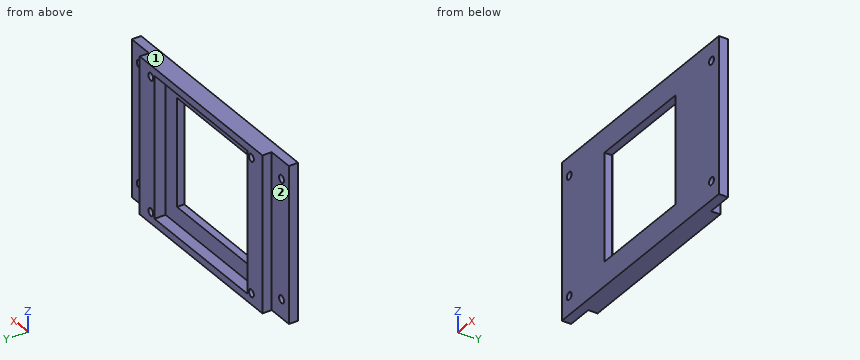
```python
from build123d import *

# Parameters (mm, degrees)
SKETCH1_R            = 11
SKETCH1_R_2          = 7.5
EXTRUDE_THIN1_DEPTH  = 10
BOSS_EXTRUDE2_DEPTH  = 10
SKETCH6_W            = 10
SKETCH6_H            = 5
BOSS_EXTRUDE3_DEPTH  = 10
SKETCH8_W            = 10
SKETCH8_H            = 5
BOSS_EXTRUDE4_DEPTH  = 10
SKETCH9_W            = 42
SKETCH9_H            = 5
BOSS_EXTRUDE5_DEPTH  = 54
SKETCH19_W           = 38
SKETCH19_H           = 38
CUT_EXTRUDE3_DEPTH   = 3
SKETCH25_W           = 29
SKETCH25_H           = 29
CUT_EXTRUDE4_DEPTH   = 2
SKETCH26_R           = 1.00264766
CUT_EXTRUDE5_DEPTH   = 3
LPATTERN4_COUNT      = 2
LPATTERN4_PITCH      = 36
LPATTERN4_COUNT_DIR2 = 2
LPATTERN4_PITCH_DIR2 = 41
SKETCH29_W           = 22
SKETCH29_H           = 36
CUT_EXTRUDE8_DEPTH   = 10
SKETCH35_R           = 1
CUT_EXTRUDE9_DEPTH   = 5
LPATTERN5_COUNT      = 2
LPATTERN5_PITCH      = 58
LPATTERN5_COUNT_DIR2 = 2
LPATTERN5_PITCH_DIR2 = 32
SKETCH37_W           = 42
SKETCH37_H           = 2.5
CUT_EXTRUDE10_DEPTH  = 5
SKETCH38_W           = 42
SKETCH38_H           = 2.5
CUT_EXTRUDE11_DEPTH  = 5
SKETCH39_W           = 1.998284703
SKETCH39_H           = 42
CUT_EXTRUDE12_DEPTH  = 2.5
SKETCH41_W           = 1.997921913
SKETCH41_H           = 42
CUT_EXTRUDE13_DEPTH  = 2.5


with BuildPart() as part:
    # Sketch1 → Extrude-Thin1 (new body)
    with BuildSketch(Plane(origin=(0, 0, 0), x_dir=(0, 0, -1), z_dir=(1, 0, 0))):
        Circle(SKETCH1_R)
        Circle(SKETCH1_R_2, mode=Mode.SUBTRACT)
    extrude(amount=EXTRUDE_THIN1_DEPTH)

    # Sketch3 → Boss-Extrude2 (add)
    with BuildSketch(Plane(origin=(0, 0, 0), x_dir=(0, 0, -1), z_dir=(1, 0, 0))):
        with BuildLine():
            Line((-11, 0), (-11, 30))
            Line((-11, 30), (11, 30))
            Line((11, 30), (11, 0))
            ThreePointArc((11, 0), (0, 11), (-11, 0))
        make_face()
    extrude(amount=BOSS_EXTRUDE2_DEPTH)

    # Sketch6 → Boss-Extrude3 (add)
    with BuildSketch(Plane.XY.offset(11)):
        with Locations((5, 27.5)):
            Rectangle(SKETCH6_W, SKETCH6_H)
    extrude(amount=BOSS_EXTRUDE3_DEPTH)

    # Sketch8 → Boss-Extrude4 (add)
    with BuildSketch(Plane(origin=(0, 0, -11), x_dir=(-1, 0, 0), z_dir=(0, 0, -1))):
        with Locations((-5, 27.5)):
            Rectangle(SKETCH8_W, SKETCH8_H)
    extrude(amount=BOSS_EXTRUDE4_DEPTH)

    # Sketch9 → Boss-Extrude5 (add)
    with BuildSketch(Plane.ZY):
        with Locations((0, 27.5)):
            Rectangle(SKETCH9_W, SKETCH9_H)
    extrude(amount=BOSS_EXTRUDE5_DEPTH)

    # Sketch19 → Cut-Extrude3 (cut)
    with BuildSketch(Plane(origin=(0, 30, 0), x_dir=(1, 0, 0), z_dir=(0, 1, 0))):
        with Locations((-22, 0)):
            Rectangle(SKETCH19_W, SKETCH19_H)
    extrude(amount=-CUT_EXTRUDE3_DEPTH, mode=Mode.SUBTRACT)

    # Sketch25 → Cut-Extrude4 (cut)
    with BuildSketch(Plane(origin=(0, 27, 0), x_dir=(1, 0, 0), z_dir=(0, 1, 0))):
        with Locations((-22.144950272, -0.049169749)):
            Rectangle(SKETCH25_W, SKETCH25_H)
    extrude(amount=-CUT_EXTRUDE4_DEPTH, mode=Mode.SUBTRACT)

    # Sketch26 → Cut-Extrude5 (cut)
    with BuildSketch(Plane(origin=(0, 30, 0), x_dir=(1, 0, 0), z_dir=(0, 1, 0))):
        with Locations(Location((-1.5, 17.99735234, 0), (0, 0, 270))):
            Circle(SKETCH26_R)
    cut_extrude5 = extrude(amount=-CUT_EXTRUDE5_DEPTH, mode=Mode.SUBTRACT)

    # LPattern4: Cut-Extrude5 2 × 2
    with Locations(*[(-j * LPATTERN4_PITCH_DIR2, 0, i * LPATTERN4_PITCH) for i in range(LPATTERN4_COUNT) for j in range(LPATTERN4_COUNT_DIR2) if (i, j) != (0, 0)]):
        add(cut_extrude5, mode=Mode.SUBTRACT)

    # Sketch29 → Cut-Extrude8 (cut)
    with BuildSketch(Plane(origin=(10, 0, 0), x_dir=(0, 0, -1), z_dir=(1, 0, 0))):
        with Locations((0, 7)):
            Rectangle(SKETCH29_W, SKETCH29_H)
    extrude(amount=-CUT_EXTRUDE8_DEPTH, mode=Mode.SUBTRACT)

    # Sketch35 → Cut-Extrude9 (cut)
    with BuildSketch(Plane(origin=(0, 30, 0), x_dir=(1, 0, 0), z_dir=(0, 1, 0))):
        with Locations(Location((7, 16, 0), (0, 0, 270))):
            Circle(SKETCH35_R)
    cut_extrude9 = extrude(amount=-CUT_EXTRUDE9_DEPTH, mode=Mode.SUBTRACT)

    # LPattern5: Cut-Extrude9 2 × 2
    with Locations(*[(-i * LPATTERN5_PITCH, 0, j * LPATTERN5_PITCH_DIR2) for i in range(LPATTERN5_COUNT) for j in range(LPATTERN5_COUNT_DIR2) if (i, j) != (0, 0)]):
        add(cut_extrude9, mode=Mode.SUBTRACT)

    # Sketch37 → Cut-Extrude10 (cut)
    with BuildSketch(Plane(origin=(10, 0, 0), x_dir=(0, 0, -1), z_dir=(1, 0, 0))):
        with Locations((0, 28.75)):
            Rectangle(SKETCH37_W, SKETCH37_H)
    extrude(amount=-CUT_EXTRUDE10_DEPTH, mode=Mode.SUBTRACT)

    # Sketch38 → Cut-Extrude11 (cut)
    with BuildSketch(Plane.ZY.offset(54)):
        with Locations((0, 28.75)):
            Rectangle(SKETCH38_W, SKETCH38_H)
    extrude(amount=-CUT_EXTRUDE11_DEPTH, mode=Mode.SUBTRACT)

    # Sketch39 → Cut-Extrude12 (cut)
    with BuildSketch(Plane(origin=(0, 30, 0), x_dir=(1, 0, 0), z_dir=(0, 1, 0))):
        with Locations((-48.000857649, 0)):
            Rectangle(SKETCH39_W, SKETCH39_H)
    extrude(amount=-CUT_EXTRUDE12_DEPTH, mode=Mode.SUBTRACT)

    # Sketch41 → Cut-Extrude13 (cut)
    with BuildSketch(Plane(origin=(0, 30, 0), x_dir=(1, 0, 0), z_dir=(0, 1, 0))):
        with Locations((4.001039044, 0)):
            Rectangle(SKETCH41_W, SKETCH41_H)
    extrude(amount=-CUT_EXTRUDE13_DEPTH, mode=Mode.SUBTRACT)


solid = part.part
```
Read the model definition and answer for the solid it produces. Units are mm, in the model's axes. Face numbers are marked on the shaded views. A direction names the side the tool comes from. Give positions to 0.01 mm unless a question says otherwise; leave off trailing zeros. Order: outer loops, then holes, each group sorted by start corner. A loop starts at its lowest first (then second) coordinate and runs counter-clockwise, first axis right, second up.
(1) Find section C-C (x = -51). Give the vertices of the cut face in (y, z).
(2) Find section A-A (z = 9.5). Give the vertices of the cut face in (x, y), plus the area to 3 significant figures.
(3) Find section D-D (z = -16). Give the vertices of the cut face in (x, y), plus the area to 3 significant figures.
(4) For the marked faces 1 and 2, determine the directions among +Z, -Z, +X, -X, +Y, -Y from which every point of the face is accessible in a straight line to the end or side of a thin tool.
(5) Straight lines are drawn through the part: L1, parallel to Z at x = -3.5, y = 28.25; L2, parallel to X at y = 28.6, z = 2; L3, parallel to Y at x = 6.5, z = -14.5. For each, find the intervals that lie inside material, in ascending order.
(6) Given pin 1 (1.6 mm diameter, centred on x = -42, z = 18, fed in from +Y); pin 2 (1.5 mm diameter, centred on y = 29, z = 9, fed in from +X); pin 3 (5.5 mm diameter, centred on x = 7.5, z = 3, fed in from +Y), each flat-ended and moving along its own axis, determine where each tip first touches the part or whether it passes through.
(7) Find section B-B (y = 25.9). Give the vertices of the cut face in (x, z).
Result sheet:
1. outline: (25, -21) - (27.5, -21) - (27.5, -17) - (25, -17) - close; (25, -15) - (27.5, -15) - (27.5, 15) - (25, 15) - close; (25, 17) - (27.5, 17) - (27.5, 21) - (25, 21) - close
2. outline: (-54, 25) - (-36.64, 25) - (-36.64, 27) - (-41, 27) - (-41, 30) - (-47, 30) - (-47, 27.5) - (-54, 27.5) - close; (-7.64, 25) - (10, 25) - (10, 27.5) - (3, 27.5) - (3, 30) - (-3, 30) - (-3, 27) - (-7.64, 27) - close
2. area: 113 mm2
3. outline: (-54, 25) - (-52, 25) - (-52, 27.5) - (-54, 27.5) - close; (-50, 25) - (6, 25) - (6, 27.5) - (3, 27.5) - (3, 30) - (-3, 30) - (-3, 27) - (-41, 27) - (-41, 30) - (-47, 30) - (-47, 27.5) - (-50, 27.5) - close; (8, 25) - (10, 25) - (10, 27.5) - (8, 27.5) - close
3. area: 161 mm2
4. face 1: +Z, +X, -X, +Y, -Y
4. face 2: +Z, -Z, -X, +Y
5. L1: z = -21 to -19, 19 to 21
5. L2: x = -47 to -41, -3 to 3
5. L3: y = 25 to 27.5
6. pin 1: stops at y = 30
6. pin 2: stops at x = 3
6. pin 3: stops at y = 27.5
7. outline: (-54, -21) - (10, -21) - (10, 21) - (-54, 21) - close; hole circle Ø2 at (-51, -16); hole circle Ø2 at (-51, 16); hole (-36.64, -14.45) - (-7.64, -14.45) - (-7.64, 14.55) - (-36.64, 14.55) - close; hole circle Ø2 at (7, -16); hole circle Ø2 at (7, 16)
